Read the model definition and answer for the solid it produces. Units are mm, in the model's axes. Face numbers are marked on the shaded views. A direction names the side the tool comes from. Coordinates: 2 decimals unless noted, no trailing zeros. Write each loop counter-clockwise with the first axis right and the second up, starting at its lowest first coordinate (ties: lowest second). Pieces come first, ordered by that corner, then holes.
1) Each of these flat-tipped pins is pushed along its axis until it touches: pin 1 Ø1.3 at (x, y) = (-1, -1) entering from -Z; pin 2 Ø2 at (x, y) = (0, -3) entering from -Z. Where does it stop, or does it pass through?
2) The part is cut by section C-C (z = 5.5). Determine the outline of the cut face in (x, y), then the cut area to 3 significant figures.
3) Determine the mould class of the marked faces 3, 4 and 5 for opening direction X: +X half, -X half, draft (parallel to the pull), parting line (faces both ways), or undercut.
4) The part is cut by section A-A (x = 0). Determine the outline of the cut face in (y, z).
5) The part is cut by section D-D (x = -3). Determine the outline of the cut face in (y, z).
6) Find the intervals of material crossed by line 1 (Z direction, x = 2.5, y = 2); line 2 (X direction, y = 0, z = 21.75); line 3 (Z direction, x = -1.5, y = -1.5), in increasing order.
7) Which of the six approach directions +Z, -Z, +X, -X, +Y, -Y give full straight-line access (tool end or side, diameter ignored) to the marked faces 1 and 2?
8) The part is cut by section B-B (y = -1.5). Determine the outline of the cut face in (x, z).
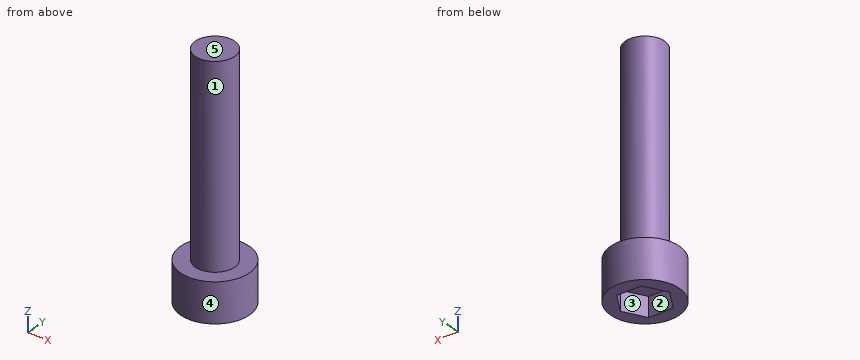
from build123d import *

# Parameters (mm, degrees)
POCKET_DEPTH = 2


with BuildPart() as part:
    # Sketch → Revolution (revolve)
    with BuildSketch(Plane.YZ):
        Polygon((-3.5, 4), (-3.5, 0), (0, 0), (0, 24), (-2, 24), (-2, 4), align=None)
    revolve(axis=Axis((0, 0, 0), (0, 0, 1)))

    # Sketch001 (on Face2 of Revolution) → Pocket (cut)
    with BuildSketch(Plane.YX):
        Polygon((0, 2.5), (-2.165064, 1.25), (-2.165064, -1.25), (0, -2.5), (2.165064, -1.25), (2.165064, 1.25), align=None)
    extrude(amount=-POCKET_DEPTH, mode=Mode.SUBTRACT)


solid = part.part
Reported:
1. pin 1: stops at z = 2
1. pin 2: stops at z = 0
2. outline: circle Ø4 at (0, 0)
2. area: 12.6 mm2
3. face 3: undercut
3. face 4: parting line
3. face 5: draft
4. outline: (-3.5, 0) - (-2.17, 0) - (-2.17, 2) - (2.17, 2) - (2.17, 0) - (3.5, 0) - (3.5, 4) - (2, 4) - (2, 24) - (-2, 24) - (-2, 4) - (-3.5, 4) - close
5. outline: (-1.8, 0) - (1.8, 0) - (1.8, 4) - (-1.8, 4) - close
6. line 1: z = 0 to 4
6. line 2: x = -2 to 2
6. line 3: z = 2 to 4
7. face 1: +Z
7. face 2: -Z
8. outline: (-3.16, 0) - (-1.63, 0) - (-1.63, 2) - (1.63, 2) - (1.63, 0) - (3.16, 0) - (3.16, 4) - (1.32, 4) - (1.32, 24) - (-1.32, 24) - (-1.32, 4) - (-3.16, 4) - close
